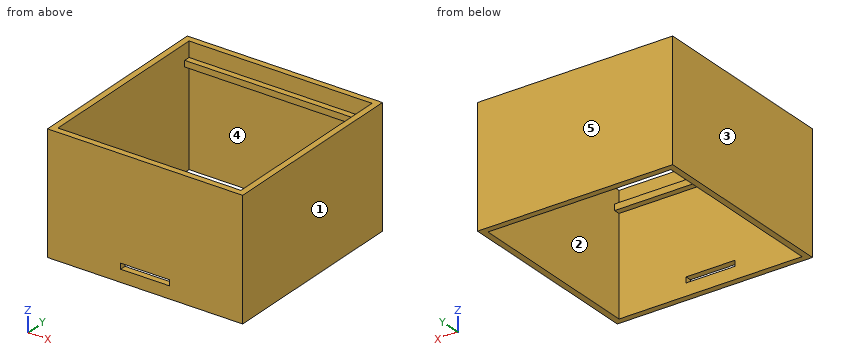
```python
from build123d import *

# Parameters (mm, degrees)
F1_DEPTH = 123.825
F2_W     = 190.5
F2_H     = 6.35
F3_DEPTH = 6.35
F4_W     = 190.5
F4_H     = 6.35
F5_DEPTH = 6.35
F7_DEPTH = 25.4


with BuildPart() as f1:
    # F0 (on Top) → F1 (new body)
    with BuildSketch(Plane.XY):
        Polygon((101.6, -101.6), (101.6, 101.6), (95.25, 95.25), (95.25, -95.25), align=None)
        Polygon((-95.25, -95.25), (-101.6, -101.6), (101.6, -101.6), (95.25, -95.25), align=None)
        Polygon((-95.25, 95.25), (-101.6, 101.6), (-101.6, -101.6), (-95.25, -95.25), align=None)
        Polygon((101.6, 101.6), (-101.6, 101.6), (-95.25, 95.25), (95.25, 95.25), align=None)
    extrude(amount=F1_DEPTH)

    # F2 (on face) → F3 (join)
    with BuildSketch(Plane.XZ.offset(-95.25)):
        with Locations((0, 104.775)):
            Rectangle(F2_W, F2_H)
    extrude(amount=F3_DEPTH)

    # F4 (on face) → F5 (join)
    with BuildSketch(Plane(origin=(0, -95.25, 0), x_dir=(-1, 0, 0), z_dir=(0, 1, 0))):
        with Locations((0, 104.775)):
            Rectangle(F4_W, F4_H)
    extrude(amount=F5_DEPTH)

    # F6 (on face) → F7 (cut)
    with BuildSketch(Plane.XZ.offset(101.6)):
        Polygon((-25.4, 12.7), (0, 12.7), (25.4, 12.7), (25.4, 18.542), (-25.4, 18.542), align=None)
    extrude(amount=-F7_DEPTH, mode=Mode.SUBTRACT)


solid = f1.part
```
For this review, take the finished solid that the model builds, in its own axes (mm). Face numbers are marked on the shaded views. A direction names the side the tool comes from. Round coordinates to 2 decimals unless told otherwise and drop trailing zeros. Write each loop counter-clockwise with the first axis right and the second up, starting at its lowest first coordinate (ties: lowest second). Pieces come first, ordered by that corner, then holes. Notation, with made-up numbers: (-22, 7) - (11, 7) arc R16 ccw to (11, 31) - close; hole circle Ø6 at (66, 6.5). An arc over 180 degrees is marked (long way). Answer as a JSON object with one key per item and string values.
1. Draft analysis for pull direction X (two halves, no side actions). For the marked faces 1, 2 and 3, state which applies: +X half, -X half, draft (parallel to the pull), parting line (faces both ways), or undercut.
Response values:
{"face 1": "+X half", "face 2": "undercut", "face 3": "-X half"}
2. We need section A-A on x = -13. Give the boundary of the cut face in (y, z) (3 decimals), then the cut area to 3 significant figures.
Response values:
{"outline": "(-101.6, 0) - (-95.25, 0) - (-95.25, 12.7) - (-101.6, 12.7) - close; (-101.6, 18.542) - (-95.25, 18.542) - (-95.25, 101.6) - (-88.9, 101.6) - (-88.9, 107.95) - (-95.25, 107.95) - (-95.25, 123.825) - (-101.6, 123.825) - close; (88.9, 101.6) - (95.25, 101.6) - (95.25, 0) - (101.6, 0) - (101.6, 123.825) - (95.25, 123.825) - (95.25, 107.95) - (88.9, 107.95) - close", "area": "1,620 mm2"}
3. To check wall thickness, follow line 1 along X through (y, z) = (-54.5, 89.5); line 2 along Y through (x, z) = (27.5, 103.5). State the ranges of each line that lie inside material, in increasing order.
Response values:
{"line 1": "x = -101.6 to -95.25, 95.25 to 101.6", "line 2": "y = -101.6 to -88.9, 88.9 to 101.6"}
4. For pin 1 Ø1.9 at (x, y) = (-5, -91.5) entering from +Z; pin 2 Ø5 at (x, y) = (33, -90.5) entering from -Z, all flat-tipped, find the tip position at first contact; note any pin that passes through.
Response values:
{"pin 1": "stops at z = 107.95", "pin 2": "stops at z = 101.6"}
5. We need section B-B on y = -28. Give the boundary of the cut face in (x, z) (3 decimals), then the cut area to 3 significant figures.
Response values:
{"outline": "(-101.6, 0) - (-95.25, 0) - (-95.25, 123.825) - (-101.6, 123.825) - close; (95.25, 0) - (101.6, 0) - (101.6, 123.825) - (95.25, 123.825) - close", "area": "1,570 mm2"}
6. We need section D-D on z = 72. Give the boundary of the cut face in (x, y), then the cut area to 3 significant figures.
Response values:
{"outline": "(-101.6, -101.6) - (101.6, -101.6) - (101.6, 101.6) - (-101.6, 101.6) - close; hole (-95.25, -95.25) - (95.25, -95.25) - (95.25, 95.25) - (-95.25, 95.25) - close", "area": "5,000 mm2"}
7. We need section C-C on x = -64. Give the boundary of the cut face in (y, z) (3 decimals), then the cut area to 3 significant figures.
Response values:
{"outline": "(-101.6, 0) - (-95.25, 0) - (-95.25, 101.6) - (-88.9, 101.6) - (-88.9, 107.95) - (-95.25, 107.95) - (-95.25, 123.825) - (-101.6, 123.825) - close; (88.9, 101.6) - (95.25, 101.6) - (95.25, 0) - (101.6, 0) - (101.6, 123.825) - (95.25, 123.825) - (95.25, 107.95) - (88.9, 107.95) - close", "area": "1,650 mm2"}
8. Tool access review of the marked faces 4 and 5: name each direction out of +Z, -Z, +X, -X, +Y, -Y from which nothing blocks a thin tool from reaching the whole face with its end or side.
Response values:
{"face 4": "-Z", "face 5": "+Z, -Z, +X, -X, +Y"}
